```python
from build123d import *

# Parameters (mm, degrees)
SKETCH2_W               = 56.896
SKETCH2_H               = 18.0086
BOSS_EXTRUDE1_DEPTH     = 9.9949
SKETCH3_R               = 4.01574
SKETCH3_R_2             = 4.50596
CUT_EXTRUDE1_DEPTH      = 10.0043
CUT_EXTRUDE1_DEPTH_BACK = 10.0043
SKETCH5_OUTSIDE_W       = 71.484
SKETCH5_OUTSIDE_H       = 34.578
CUT_EXTRUDE2_DEPTH      = 10.0043
CUT_EXTRUDE2_DEPTH_BACK = 10.0043
CUT_EXTRUDE3_DEPTH      = 10.0043
CUT_EXTRUDE3_DEPTH_BACK = 10.0043
FILLET1_R               = 4.7752
SKETCH7_W               = 16.002
SKETCH7_H               = 10.1092
CUT_EXTRUDE4_DEPTH      = 10.9949
CUT_EXTRUDE4_DEPTH_BACK = 10.9949


with BuildPart() as part:
    # Sketch2 → Boss-Extrude1 (new body, symmetric)
    with BuildSketch(Plane(origin=(0, 0, 0), x_dir=(1, 0, 0), z_dir=(0, 1, 0))):
        Rectangle(SKETCH2_W, SKETCH2_H)
    extrude(amount=BOSS_EXTRUDE1_DEPTH, both=True)

    # Sketch3 → Cut-Extrude1 (cut, two sides)
    with BuildSketch(Plane.XY) as cut_extrude1_sk:
        with Locations((21.9456, -1.0033)):
            Circle(SKETCH3_R)
        with Locations((0.2032, 1.0033)):
            Circle(SKETCH3_R_2)
    extrude(amount=CUT_EXTRUDE1_DEPTH, mode=Mode.SUBTRACT)
    extrude(cut_extrude1_sk.sketch, amount=-CUT_EXTRUDE1_DEPTH_BACK, mode=Mode.SUBTRACT)

    # Sketch5 outside → Cut-Extrude2 (cut, two sides)
    with BuildSketch(Plane.XY) as cut_extrude2_sk:
        Rectangle(SKETCH5_OUTSIDE_W, SKETCH5_OUTSIDE_H)
        with BuildLine():
            Line((18.049040748, -9.9949), (24.693632985, -6.896475754))
            ThreePointArc((24.693632985, -6.896475754), (27.429668537, -4.497036973), (28.448, -1.0033))
            Line((28.448, -1.0033), (28.448, -0.818554854))
            ThreePointArc((28.448, -0.818554854), (27.509225683, 2.402233918), (24.986942908, 4.614216544))
            Line((24.986942908, 4.614216544), (13.44803, 9.9949))
            Line((13.44803, 9.9949), (-1.778, 9.9949))
            Line((-1.778, 9.9949), (-28.448, -2.441525243))
            Line((-28.448, -2.441525243), (-28.448, -9.9949))
            Line((-28.448, -9.9949), (18.049040748, -9.9949))
        make_face(mode=Mode.SUBTRACT)
    extrude(amount=CUT_EXTRUDE2_DEPTH, mode=Mode.SUBTRACT)
    extrude(cut_extrude2_sk.sketch, amount=-CUT_EXTRUDE2_DEPTH_BACK, mode=Mode.SUBTRACT)

    # Sketch6 → Cut-Extrude3 (cut, two sides)
    with BuildSketch(Plane.XY) as cut_extrude3_sk:
        with BuildLine():
            Line((-5.7912, -9.9949), (-8.7884, -6.9977))
            Line((-8.7884, -6.9977), (-16.175422135, -6.9977))
            ThreePointArc((-16.175422135, -6.9977), (-22.178675052, -9.492417259), (-28.448, -7.772468279))
            Line((-28.448, -7.772468279), (-28.448, -9.9949))
            Line((-28.448, -9.9949), (-5.7912, -9.9949))
        make_face()
    extrude(amount=CUT_EXTRUDE3_DEPTH, mode=Mode.SUBTRACT)
    extrude(cut_extrude3_sk.sketch, amount=-CUT_EXTRUDE3_DEPTH_BACK, mode=Mode.SUBTRACT)

    # Fillet1
    fillet1_edges = [part.edges().sort_by_distance(p)[0] for p in [
        (-16.175422135, -6.9977, 0),
        (-8.7884, -6.9977, 0),
        (-5.7912, -9.9949, 0),
    ]]
    fillet(fillet1_edges, radius=FILLET1_R)

    # Sketch7 → Cut-Extrude4 (cut, two sides)
    with BuildSketch(Plane(origin=(0, 0, 0), x_dir=(1, 0, 0), z_dir=(0, 1, 0))) as cut_extrude4_sk:
        with Locations((20.447, 0)):
            Rectangle(SKETCH7_W, SKETCH7_H)
    extrude(amount=CUT_EXTRUDE4_DEPTH, mode=Mode.SUBTRACT)
    extrude(cut_extrude4_sk.sketch, amount=-CUT_EXTRUDE4_DEPTH_BACK, mode=Mode.SUBTRACT)


solid = part.part
```
Input: part model. Units: mm. Frame: model coordinates. A direction names the side the tool comes from. Give positions to 0.01 mm unless a question says otherwise; leave off trailing zeros. Order: outer loops, then holes, each group sorted by start corner. A loop starts at its lowest first (then second) coordinate and runs counter-clockwise, first axis right, second up. Notation, with made-up numbers: (44, 50.25) - (88, 50.25) arc R18 ccw to (88, 68.25) - close; hole circle Ø3 at (55, -7.75). An arc over 180 degrees is marked (long way). One line per item, written item: value.
1. Line query: probe 1 along Z at (x, y) = (15, -0.5); probe 2 along X at (y, z) = (0.5, -7); probe 3 along X at (y, z) = (-8.25, -4.5). Output: solid intervals per line, ascending.
Determined:
probe 1: -9 to -5.05, 5.05 to 9
probe 2: -22.14 to -4.27, 4.68 to 18.22, 25.67 to 28.3
probe 3: -27.67 to -17.94, -7.54 to 12.45
2. Cut plane B-B, the plane x = 19. Output: boundary loops of the cut face in (y, z), and give its area (3 significant figures).
Determined:
outline: (-9.55, -9) - (-3.73, -9) - (-3.73, -5.05) - (-9.55, -5.05) - close; (-9.55, 5.05) - (-3.73, 5.05) - (-3.73, 9) - (-9.55, 9) - close; (1.73, -9) - (7.41, -9) - (7.41, -5.05) - (1.73, -5.05) - close; (1.73, 5.05) - (7.41, 5.05) - (7.41, 9) - (1.73, 9) - close
area: 90.8 mm2
3. Cut plane C-C, the plane z = 1. Output: boundary loops of the cut face in (x, y).
Determined:
outline: (-28.45, -7.77) arc R10.01 ccw to (-17.23, -7.81) arc R4.78 cw to (-14.56, -7) - (-10.77, -7) arc R4.78 cw to (-7.39, -8.4) - (-7.19, -8.6) arc R4.78 ccw to (-3.81, -9.99) - (12.45, -9.99) - (12.45, 9.99) - (-1.78, 9.99) - (-28.45, -2.44) - close; hole circle Ø9.01 at (0.2, 1)
4. Pin query (flat end, axial travel): pin 1 Ø2 at (y, z) = (-1, -1) entering from +X; pin 2 Ø1 at (x, z) = (18, 7) entering from +Y; pin 3 Ø6 at (x, z) = (-8.5, 5) entering from -Y. Return the tip coordinate at first contact, or that it passes through.
Determined:
pin 1: x = 12.45
pin 2: y = 8.11
pin 3: y = -9.69
5. Cut plane D-D, the plane z = -5.75. Output: boundary loops of the cut face in (x, y).
Determined:
outline: (-28.45, -7.77) arc R10.01 ccw to (-17.23, -7.81) arc R4.78 cw to (-14.56, -7) - (-10.77, -7) arc R4.78 cw to (-7.39, -8.4) - (-7.19, -8.6) arc R4.78 ccw to (-3.81, -9.99) - (18.05, -9.99) - (24.69, -6.9) arc R6.5 ccw to (28.45, -1) - (28.45, -0.82) arc R5.99 ccw to (24.99, 4.61) - (13.45, 9.99) - (-1.78, 9.99) - (-28.45, -2.44) - close; hole circle Ø9.01 at (0.2, 1); hole circle Ø8.03 at (21.95, -1)
6. Draft query along Z for faces 1 (the face through (17, 0, 5.055)), 2 (the face through (17, 0, -5.055)), 3 (the face through (0, -4, 9.004)), 4 (the face through (-5.62, -9.64, -0.13)). Return one class per face: released by +Z, released by -Z, zero draft, split by the parting line, or undercut.
Determined:
face 1: undercut
face 2: undercut
face 3: released by +Z
face 4: zero draft
7. Cut plane A-A, the plane y = 2. Output: boundary loops of the cut face in (x, z).
Determined:
outline: (-18.92, -9) - (-4.19, -9) - (-4.19, 9) - (-18.92, 9) - close; (4.6, -9) - (19.28, -9) - (19.28, -5.05) - (12.45, -5.05) - (12.45, 5.05) - (19.28, 5.05) - (19.28, 9) - (4.6, 9) - close; (24.61, -9) - (27.74, -9) - (27.74, -5.05) - (24.61, -5.05) - close; (24.61, 5.05) - (27.74, 5.05) - (27.74, 9) - (24.61, 9) - close
8. Reachability of faces 5 (the face through (27.535, 2.362, -7.057)), 6 (the face through (-15.94, -7.2, 0.13)) from +Z, -Z, +X, -X, +Y, -Y: full face, straight path, thin tool, end or side. Return the list, or none.
Determined:
face 5: +Z, -Z, +X, +Y
face 6: +Z, -Z, -Y
